Design review of the part built by this model. Coordinates are the model's own, in mm. A direction names the side the tool comes from. Coordinates: 2 decimals unless noted, no trailing zeros. Loops run counter-clockwise (first coordinate to the right, second up) from the corner with the lowest first, then second, coordinate; pieces in that order, holes last. Notation, with made-up numbers: M 6.5,3 L 51.5,3 A10 ccw 51.5,19 Z; hole C -30,34.5 d10. An arc over 180 degrees is marked long. Answer as a JSON object with one key per item and string values. Group by question number.
1. Machinability: for faces 1 (the flat face through (11.5, -3, 5)), 2 (the flat face through (22, -11, 0)), 3 (the flat face through (-15, 4, -6)), which of the approach directions +Z, -Z, +X, -X, +Y, -Y give a long, thin tool a straight path to every point of the face, cutting with its end or side? Answer none if there is none.
2. Consider section C-C (x = 0). State the section outline as (y, z) points, then the cut area to 3 significant figures.
3. Draft analysis for pull direction X (two halves, no side actions). For faces 4 (the flat face through (11.5, -3, 29)), 5 (the flat face through (0, 13, 33)), 6 (the flat face through (0, 13, 0)), 7 (the flat face through (-30, 3, 3)), state which applies: +X half, -X half, draft (parallel to the pull), parting line (faces both ways), or undercut.
4. Consider section A-A (y = -5). State the section outline as (x, z) points.
5. Consider section B-B (z = -2.5). State the section outline as (x, y) points.
6. Insertion check: pin 1 (8 mm diameter, centred on y = -10.5, z = 22.5, fed in from +X); pin 2 (25 mm diameter, centred on x = 0, z = 18, fed in from -Y); pin 3 (1 mm diameter, centred on x = 13, z = 13, fed in from -Y); pin 4 (11 mm diameter, centred on x = 21.5, y = -13, fed in from -Z). Each pin has a flat end and moves straight along its axis. Give the tip position at first contact, or say it passes through.
7. To check wall thickness, follow probe 1 along X at (y, z) = (1.25, -6); probe 2 along Z at (x, y) = (24, 0.25); probe 3 along X at (y, z) = (-10.5, 12). State the ranges of each line that lie inside material, in increasing order.
8. Consider section D-D (y = 9.5). State the section outline as (x, z) points, then the cut area to 3 significant figures.
from build123d import *

# Parameters (mm, degrees)
BOSS_EXTRUDE1_DEPTH = 33
SKETCH3_R           = 14
CUT_EXTRUDE1_DEPTH  = 21
SKETCH4_W           = 15
SKETCH4_H           = 45
BOSS_EXTRUDE2_DEPTH = 20
SKETCH7_W           = 15
SKETCH7_H           = 33
BOSS_EXTRUDE3_DEPTH = 10
FILLET1_R           = 15


with BuildPart() as part:
    # Sketch2 → Boss-Extrude1 (new body)
    with BuildSketch(Plane.XY):
        with BuildLine():
            Line((11.5, 0), (11.5, -6))
            Line((11.5, -6), (15, -6))
            Line((15, -6), (15, 14))
            Line((15, 14), (-15, 14))
            Line((-15, 14), (-15, -6))
            Line((-15, -6), (-11.5, -6))
            Line((-11.5, -6), (-11.5, 0))
            ThreePointArc((-11.5, 0), (0, 11.5), (11.5, 0))
        make_face()
    extrude(amount=BOSS_EXTRUDE1_DEPTH)

    # Sketch3 → Cut-Extrude1 (cut, through all)
    with BuildSketch(Plane(origin=(0, 14, 0), x_dir=(1, 0, 0), z_dir=(0, 1, 0))):
        with Locations((0, -18)):
            Circle(SKETCH3_R)
    extrude(amount=-CUT_EXTRUDE1_DEPTH, mode=Mode.SUBTRACT)

    # Sketch4 → Boss-Extrude2 (add)
    with BuildSketch(Plane(origin=(0, 14, 0), x_dir=(1, 0, 0), z_dir=(0, 1, 0))):
        with Locations((22.5, -10.5)):
            Rectangle(SKETCH4_W, SKETCH4_H)
    boss_extrude2 = extrude(amount=-BOSS_EXTRUDE2_DEPTH)

    # Sketch6 → M5x0.8 Tapped Hole1 (revolve, cut)
    with BuildSketch(Plane(origin=(24, -6, -6), x_dir=(0, 0, -1), z_dir=(1, 0, 0))):
        Polygon((0, 0), (0, 13.6618073), (2.1, 12.4), (2.1, 0), align=None)
    m5x0_8_tapped_hole1 = revolve(axis=Axis((24, -12.35, -6), (0, 1, 0)), mode=Mode.SUBTRACT)

    # Sketch7 → Boss-Extrude3 (add)
    with BuildSketch(Plane.XZ.offset(6)):
        with Locations((22.5, 16.5)):
            Rectangle(SKETCH7_W, SKETCH7_H)
    boss_extrude3 = extrude(amount=BOSS_EXTRUDE3_DEPTH)

    # Mirror1: Boss-Extrude2, M5x0.8 Tapped Hole1, Boss-Extrude3 across plane
    add(boss_extrude2.mirror(Plane(origin=(0, 0, 0), x_dir=(0, 0, 1), z_dir=(1, 0, 0))))
    add(m5x0_8_tapped_hole1.mirror(Plane(origin=(0, 0, 0), x_dir=(0, 0, 1), z_dir=(1, 0, 0))), mode=Mode.SUBTRACT)
    add(boss_extrude3.mirror(Plane(origin=(0, 0, 0), x_dir=(0, 0, 1), z_dir=(1, 0, 0))))

    # Fillet1
    fillet1_edges = [part.edges().sort_by_distance(p)[0] for p in [
        (30, -1, 33),
        (-30, -1, 33),
    ]]
    fillet(fillet1_edges, radius=FILLET1_R)


solid = part.part
Findings below:
{
 "1": {"face 1": "+Z, -Z, -Y", "face 2": "-Z, +X, -X, -Y", "face 3": "-Z, +Y, -Y"},
 "2": {"outline": "M 11.5,0 L 14,0 L 14,4 L 11.5,4 Z; M 11.5,32 L 14,32 L 14,33 L 11.5,33 Z", "area": "12.5 mm^2"},
 "3": {"face 4": "undercut", "face 5": "draft", "face 6": "undercut", "face 7": "-X half"},
 "4": {"outline": "M -30,-12 L -15,-12 L -15,0 L -11.5,0 L -11.5,10.02 A14 cw -11.5,25.98 L -11.5,33 L -15,33 A15 ccw -30,18 Z; M 11.5,0 L 15,0 L 15,-12 L 30,-12 L 30,18 A15 ccw 15,33 L 11.5,33 L 11.5,25.98 A14 cw 11.5,10.02 Z; hole C -24,-6 d4.2; hole C 24,-6 d4.2"},
 "5": {"outline": "M -30,-6 L -15,-6 L -15,14 L -30,14 Z; M 15,-6 L 30,-6 L 30,14 L 15,14 Z"},
 "6": {"pin 1": "stops at x = 29.99", "pin 2": "passes through", "pin 3": "stops at y = -6", "pin 4": "stops at z = 0"},
 "7": {"probe 1": "x = -30 to -26.1, -21.9 to -15, 15 to 21.9, 26.1 to 30", "probe 2": "z = -12 to -8.1, -3.9 to 30", "probe 3": "x = -30 to -15, 15 to 30"},
 "8": {"outline": "M -30,-12 L -15,-12 L -15,0 L -6.48,0 L -6.48,5.59 A14 cw -6.48,30.41 L -6.48,33 L -15,33 A15 ccw -30,18 Z; M 6.48,0 L 15,0 L 15,-12 L 30,-12 L 30,18 A15 ccw 15,33 L 6.48,33 L 6.48,30.41 A14 cw 6.48,5.59 Z", "area": "1,550 mm^2"}
}
